Read the model definition and answer for the solid it produces. Units are mm, in the model's axes. A direction names the side the tool comes from. Give positions to 0.01 mm unless a question says otherwise; leave off trailing zeros. Order: outer loops, then holes, each group sorted by start corner. A loop starts at its lowest first (then second) coordinate and runs counter-clockwise, first axis right, second up. Notation, with made-up numbers: (17, -39) - (53, -39) arc R9 ccw to (53, -31) - close; hole circle Ø4 at (-8.5, 9). An arc over 180 degrees is marked (long way). Write item = value, one per line.
```python
from build123d import *
from build123d.topology import SkipClean

# Parameters (mm, degrees)
CROQUIS1_R               = 95
SALIENTE_EXTRUIR1_DEPTH  = 10
CROQUIS3_R               = 95
CROQUIS3_R_2             = 91
SALIENTE_EXTRUIR2_DEPTH  = 60
SALIENTE_EXTRUIR10_DEPTH = 10
SALIENTE_EXTRUIR15_START = -10
CROQUIS7_R               = 91
CROQUIS7_R_2             = 85
SALIENTE_EXTRUIR15_DEPTH = 10


with BuildPart() as part:
    # Croquis1 → Saliente-Extruir1 (new body)
    with BuildSketch(Plane(origin=(0, 0, 0), x_dir=(1, 0, 0), z_dir=(0, 1, 0))):
        with Locations(Location((0, 0, 0), (0, 0, 270))):
            Circle(CROQUIS1_R)
    extrude(amount=SALIENTE_EXTRUIR1_DEPTH)

    # Croquis3 → Saliente-Extruir2 (add)
    with BuildSketch(Plane(origin=(0, 10, 0), x_dir=(1, 0, 0), z_dir=(0, 1, 0))):
        with Locations(Location((0, 0, 0), (0, 0, 270))):
            Circle(CROQUIS3_R)
        with Locations(Location((0, 0, 0), (0, 0, 270))):
            Circle(CROQUIS3_R_2, mode=Mode.SUBTRACT)
    extrude(amount=SALIENTE_EXTRUIR2_DEPTH)

    # Croquis4 → Saliente-Extruir10 (add)
    with BuildSketch(Plane(origin=(0, 60, 0), x_dir=(1, 0, 0), z_dir=(0, 1, 0))):
        with BuildLine():
            Line((-81.487149685, -24.183557146), (-86.820218408, -27.262605809))
            ThreePointArc((-86.820218408, -27.262605809), (-78.808311744, -45.5), (-67.020218408, -61.557211799))
            Line((-67.020218408, -61.557211799), (-61.687149685, -58.478163136))
            ThreePointArc((-61.687149685, -58.478163136), (-73.612159322, -42.5), (-81.487149685, -24.183557146))
        make_face()
        with BuildLine():
            Line((61.687149685, -58.478163136), (67.020218408, -61.557211799))
            ThreePointArc((67.020218408, -61.557211799), (78.808311744, -45.5), (86.820218408, -27.262605809))
            Line((86.820218408, -27.262605809), (81.487149685, -24.183557146))
            ThreePointArc((81.487149685, -24.183557146), (73.612159322, -42.5), (61.687149685, -58.478163136))
        make_face()
        with BuildLine():
            ThreePointArc((19.8, 88.819817608), (0, 91), (-19.8, 88.819817608))
            Line((-19.8, 88.819817608), (-19.8, 82.661720282))
            ThreePointArc((-19.8, 82.661720282), (0, 85), (19.8, 82.661720282))
            Line((19.8, 82.661720282), (19.8, 88.819817608))
        make_face()
    extrude(amount=SALIENTE_EXTRUIR10_DEPTH)

    # Croquis7 → Saliente-Extruir15 (add)
    with SkipClean():  # the faces are left unmerged after this step: merging them gives an invalid solid
        with BuildSketch(Plane(origin=(0, 60, 0), x_dir=(1, 0, 0), z_dir=(0, 1, 0)).offset(SALIENTE_EXTRUIR15_START)):
            with Locations(Location((0, 0, 0), (0, 0, 270))):
                Circle(CROQUIS7_R)
            with Locations(Location((0, 0, 0), (0, 0, 103.470293186))):
                Circle(CROQUIS7_R_2, mode=Mode.SUBTRACT)
        extrude(amount=SALIENTE_EXTRUIR15_DEPTH)


solid = part.part
```
1. For faces 1 (the face through (-19.8, 65, -86)), 2 (the face through (-70, 70, 49)), 3 (the face through (-55.372, 29.72, -72.214)), determine the directions among +Z, -Z, +X, -X, +Y, -Y from which every point of the face is accessible in a straight line to the end or side of a thin tool.
Recorded:
face_1 = +Y
face_2 = +Z, -Z, +X, -X, +Y
face_3 = none
2. Determine the mould class of faces 4 (the face through (74, 60, -44)), 5 (the face through (-92.74, 34.51, -20.59)), 6 (the face through (1, 0, -1)) for opening direction X: +X half, -X half, draft (parallel to the pull), parting line (faces both ways), or undercut.
Recorded:
face_4 = undercut
face_5 = parting line
face_6 = draft
3. Section D-D (z = 82.5) is taken. Determine the outline of the cut face in (x, y), and give its area (3 significant figures).
Recorded:
outline = (-47.1, 0) - (47.1, 0) - (47.1, 70) - (38.4, 70) - (38.4, 60) - (20.46, 60) - (20.46, 50) - (38.4, 50) - (38.4, 10) - (-38.4, 10) - (-38.4, 50) - (-20.46, 50) - (-20.46, 60) - (-38.4, 60) - (-38.4, 70) - (-47.1, 70) - close
area = 2,340 mm^2
4. Section C-C (y = 25.5) is taken. Determine the outline of the cut face in (x, z).
Recorded:
outline = circle Ø190 at (0, 0); hole circle Ø182 at (0, 0)
5. Straight lines are drawn through the part: L1, parallel to Y at x = -19, z = 85.5; L2, parallel to X at y = 57.5, z = 0; L3, parallel to X at y = 25, z = 0. For each, find the intervals that lie inside material, in ascending order. Write a range as [from, to].
Recorded:
L1 = [0, 10], [50, 60]
L2 = [-95, -85], [85, 95]
L3 = [-95, -91], [91, 95]
6. Section B-B (z = 0) is taken. Determine the outline of the cut face in (x, y), and give its area (3 significant figures).
Recorded:
outline = (-95, 0) - (95, 0) - (95, 70) - (91, 70) - (91, 60) - (85, 60) - (85, 50) - (91, 50) - (91, 10) - (-91, 10) - (-91, 50) - (-85, 50) - (-85, 60) - (-91, 60) - (-91, 70) - (-95, 70) - close
area = 2,500 mm^2
7. Section A-A (x = 0) is taken. Determine the outline of the cut face in (y, z), and give its area (3 significant figures).
Recorded:
outline = (0, -95) - (70, -95) - (70, -85) - (50, -85) - (50, -91) - (10, -91) - (10, 91) - (50, 91) - (50, 85) - (60, 85) - (60, 91) - (70, 91) - (70, 95) - (0, 95) - close
area = 2,560 mm^2
8. Flat-ended cylindrical pins translate along their axes: pin 1 (7 mm diameter, centred on y = 65, z = -87, fed in from -X); pin 2 (3 mm diameter, centred on y = 59, z = -26.5, fed in from +X); pin 3 (8 mm diameter, centred on x = -31.5, y = 40.5, fed in from +Z). Find the tip coordinate at first contact, or state that the pin passes through.
Recorded:
pin_1 = -45.31
pin_2 = 91.65
pin_3 = 90.93
